CAD build for the part. Positions are in the model's coordinates, mm. A direction names the side the tool comes from. Give positions to 0.01 mm unless a question says otherwise; leave off trailing zeros. Order: outer loops, then holes, each group sorted by start corner. A loop starts at its lowest first (then second) coordinate and runs counter-clockwise, first axis right, second up. Notation, with made-up numbers: M 30,80.25 L 67,80.25 A29 ccw 67,114.25 Z; hole C -36,-8 d7. An arc over 180 degrees is marked long. Put each result on its own line as item: value. Start each with the question number.
1) Cut at D-D (z = -1.75). Write the cut outline in (x, y).
2) Cut at B-B (x = -8.5). Write the cut outline in (y, z), and give its area (3 significant figures).
3) Tool access for faces 4 (the face through (-16, 0, 16)), 5 (the face through (-0.6, 2.96, 0.57)): list every direction of +Z, -Z, +X, -X, +Y, -Y with a clear straight run to the whole face (end or side of a thin tool).
4) Two-plate mould, pull along Z, no slides. Class faces 1 (the face through (-0.57, 2.96, 14.4)), 2 (the face through (-16, 3, 20)), 3 (the face through (-36, 3, -3)): released by +Z, released by -Z, zero draft, split by the parting line, or undercut.
5) Drill centre lines: line 1 (X direction, y = 1.55, z = 13); line 2 (Z direction, x = -2.5, y = 1.9); line 3 (X direction, y = 2.9, z = 0.5). Where is each one in solid material? Low to high. Write a range as [from, to].
6) Cut at C-C (y = 1). Write the cut outline in (x, z).
7) Cut at A-A (z = 5.5). Write the cut outline in (x, y).
Autodesk Inventor part; units mm, degrees
ref_plane "YZ Plane" through (0, 0, 0) normal (1, 0, 0) x (0, 1, 0)
ref_plane "XZ Plane" through (0, 0, 0) normal (0, 1, 0) x (-1, 0, 0)
ref_plane "XY Plane" through (0, 0, 0) normal (0, 0, 1) x (1, 0, 0)
sketch "Sketch1" plane through (0, 0, 0) normal (0, 1, 0) x (-1, 0, 0)
  line L0 (2, 0) -> (30, 0)
  line L1 (32, 2) -> (32, 13)
  line L2 (30, 15) -> (2, 15)
  line L3 (0, 13) -> (0, 2)
  line L4 (0, 20) -> (32, 20)
  line L5 (37, 15) -> (37, 0)
  line L6 (32, -5) -> (0, -5)
  line L7 (-5, 0) -> (-5, 15)
  arc A0 (0, 20) -> (-5, 15) centre (0, 15) ccw
  arc A1 (37, 15) -> (32, 20) centre (32, 15) ccw
  arc A2 (32, -5) -> (37, 0) centre (32, 0) ccw
  arc A3 (-5, 0) -> (0, -5) centre (0, 0) ccw
  arc A4 (2, 15) -> (0, 13) centre (2, 13) ccw
  arc A5 (32, 13) -> (30, 15) centre (30, 13) ccw
  arc A6 (30, 0) -> (32, 2) centre (30, 2) ccw
  arc A7 (0, 2) -> (2, 0) centre (2, 2) ccw
  point P0 (0, 0)
  point P1 (32, 0)
  point P2 (0, 15)
  dimension "d0" = 15
  dimension "d1" = 32
  dimension "d2" = 5
  dimension "d3" = 5
  dimension "d4" = 5
  dimension "d5" = 5
  dimension "d6" = 5
  dimension "d7" = 2
extrude "Extrusion1" add sketch "Sketch1" along normal blind 6
properties part number "Center Block"
Solution:
1. outline: M -36.68,0 L 4.68,0 L 4.68,6 L -36.68,6 Z
2. outline: M 0,-5 L 6,-5 L 6,0 L 0,0 Z; M 0,15 L 6,15 L 6,20 L 0,20 Z
2. area: 60.0 mm²
3. face 4: +Z, -Z, +X, -X, -Y
3. face 5: +Y, -Y
4. face 1: undercut
4. face 2: released by +Z
4. face 3: released by -Z
5. line 1: [-37, -32], [0, 5]
5. line 2: [-5, 0], [15, 20]
5. line 3: [-37, -31.32], [-0.68, 5]
6. outline: M -37,0 A5 ccw -32,-5 L 0,-5 A5 ccw 5,0 L 5,15 A5 ccw 0,20 L -32,20 A5 ccw -37,15 Z; hole M -32,2 A2 ccw -30,0 L -2,0 A2 ccw 0,2 L 0,13 A2 ccw -2,15 L -30,15 A2 ccw -32,13 Z
7. outline: M -37,0 L -32,0 L -32,6 L -37,6 Z; M 0,0 L 5,0 L 5,6 L 0,6 Z
